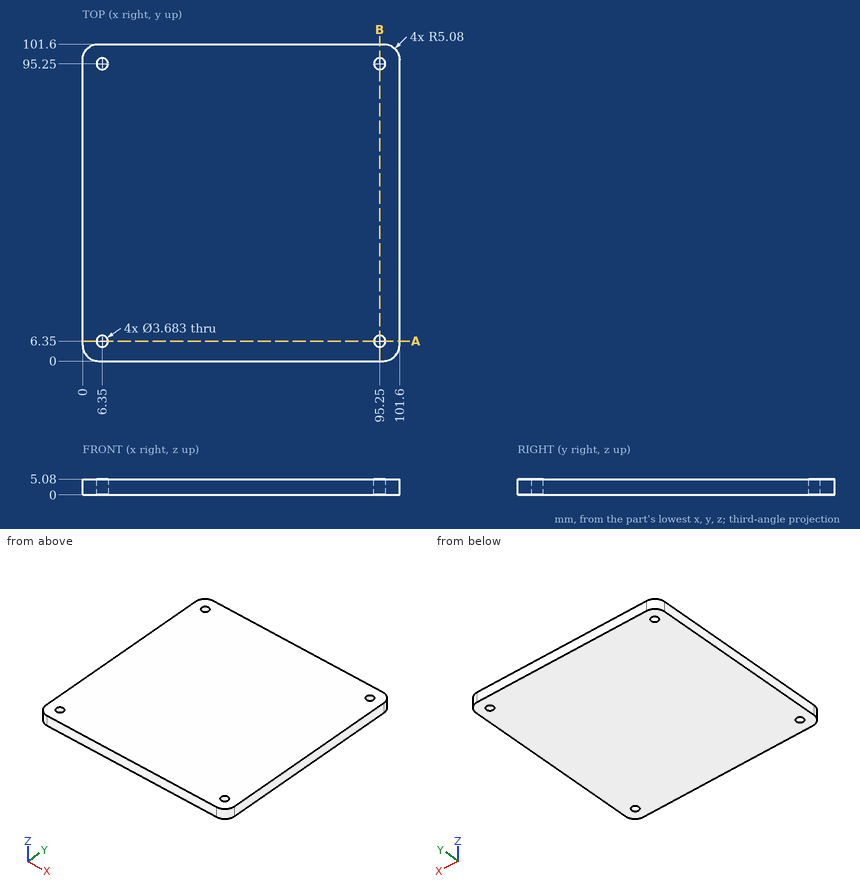
Here's the drawing with two shaded views (mm, measured from the low corner). I have some questions. Coordinates: 2 decimals unless noted, no trailing zeros. Order: outer loops, then holes, each group sorted by start corner. A loop starts at its lowest first (then second) coordinate and runs counter-clockwise, first axis right, second up.
Item 1: If we section it at A-A, the plane y = 6.35: List the corners of the cut face in (x, z) for me, then the cut area to 3 significant figures.
Response values:
outline: (0, 0) - (4.51, 0) - (4.51, 5.08) - (0, 5.08) - close; (8.19, 0) - (93.41, 0) - (93.41, 5.08) - (8.19, 5.08) - close; (97.09, 0) - (101.6, 0) - (101.6, 5.08) - (97.09, 5.08) - close
area: 479 mm2
Item 2: I'm going to push a flat-ended pin straight in: pin 1 Ø2 at (x, y) = (95.25, 6.35) entering from -Z. Where does the tip first touch, or does it pass through?
Response values:
pin 1: passes through
Item 3: I need wall thicknesses on probe 1 along Y at (x, z) = (6.35, 1.9); probe 2 along X at (y, z) = (94.5, 2.3). Which ranges of each line are inside material? Lowest first, please.
Response values:
probe 1: y = 0 to 4.51, 8.19 to 93.41, 97.09 to 101.6
probe 2: x = 0 to 4.67, 8.03 to 93.57, 96.93 to 101.6
